Verification items for the finished model (mm, model axes). A direction names the side the tool comes from. Give positions to 0.01 mm unless a question says otherwise; leave off trailing zeros. Loops run counter-clockwise (first coordinate to the right, second up) from the corner with the lowest first, then second, coordinate; pieces in that order, holes last. Notation, with made-up numbers: (81, 33.25) - (86, 33.25) arc R38 cw to (86, 71.25) - close; hole circle Ø1 at (8, 31). An arc over 180 degrees is marked (long way). Put each result on its own line as item: value. Start each with the question number.
```python
from build123d import *

# Parameters (mm, degrees)
SKETCH_1_R          = 1
EXTRUDE_1_DEPTH     = 1.6
SKETCH_2_R          = 1
CUT_EXTRUDE_1_DEPTH = 1.6
EXTRUDE_START       = 1.6
EXTRUDE_2_DEPTH     = 1.6
SKETCH_4_W          = 1.78
SKETCH_4_H          = 8.1
CUT_EXTRUDE_2_DEPTH = 0.1
CUT_EXTRUDE_START   = 1.6
SKETCH_5_W          = 1.78
SKETCH_5_H          = 8.1
CUT_EXTRUDE_3_DEPTH = 0.1
SKETCH_6_W          = 19.5
SKETCH_6_H          = 70
EXTRUDE_3_DEPTH     = 10
CUT_EXTRUDE_START_2 = 40
CUT_EXTRUDE_4_DEPTH = 70
CUT_EXTRUDE_START_3 = -10
SKETCH_9_W          = 19.5
SKETCH_9_H          = 35
CUT_EXTRUDE_5_DEPTH = 4
CUT_EXTRUDE_6_DEPTH = 1.6


with BuildPart() as part:
    # 草图1 → 凸台-拉伸1 (new body)
    with BuildSketch(Plane.XY):
        with BuildLine():
            Line((-14, 50), (14, 50))
            ThreePointArc((14, 50), (15.414213562, 49.414213562), (16, 48))
            Line((16, 48), (16, -48))
            ThreePointArc((16, -48), (15.414213562, -49.414213562), (14, -50))
            Line((14, -50), (-14, -50))
            ThreePointArc((-14, -50), (-15.414213562, -49.414213562), (-16, -48))
            Line((-16, -48), (-16, 48))
            ThreePointArc((-16, 48), (-15.414213562, 49.414213562), (-14, 50))
        make_face()
        with Locations((-14, -48)):
            Circle(SKETCH_1_R, mode=Mode.SUBTRACT)
        with Locations((14, -48)):
            Circle(SKETCH_1_R, mode=Mode.SUBTRACT)
    extrude(amount=EXTRUDE_1_DEPTH)

    # 草图2 → 切除-拉伸1 (cut)
    with BuildSketch(Plane.XY):
        with Locations((-14, 28)):
            Circle(SKETCH_2_R)
        with Locations((14, 28)):
            Circle(SKETCH_2_R)
    extrude(amount=CUT_EXTRUDE_1_DEPTH, mode=Mode.SUBTRACT)

    # 草图3 → 凸台-拉伸2 (add)
    with BuildSketch(Plane.XY.offset(EXTRUDE_START)):
        with BuildLine():
            Line((-7.62, 50), (7.62, 50))
            Line((7.62, 50), (7.62, 59.42))
            ThreePointArc((7.62, 59.42), (7.180660172, 60.480660172), (6.12, 60.92))
            Line((6.12, 60.92), (-6.12, 60.92))
            ThreePointArc((-6.12, 60.92), (-7.180660172, 60.480660172), (-7.62, 59.42))
            Line((-7.62, 59.42), (-7.62, 50))
        make_face()
        with BuildLine():
            Line((-7.62, -59.42), (-7.62, -50))
            Line((-7.62, -50), (7.62, -50))
            Line((7.62, -50), (7.62, -59.42))
            ThreePointArc((7.62, -59.42), (7.180660172, -60.480660172), (6.12, -60.92))
            Line((6.12, -60.92), (-6.12, -60.92))
            ThreePointArc((-6.12, -60.92), (-7.180660172, -60.480660172), (-7.62, -59.42))
        make_face()
    extrude(amount=-EXTRUDE_2_DEPTH)

    # 草图4 → 切除-拉伸2 (cut)
    with BuildSketch(Plane.XY):
        with Locations((0, 56.37)):
            Rectangle(SKETCH_4_W, SKETCH_4_H)
        with Locations((2.54, 56.37)):
            Rectangle(SKETCH_4_W, SKETCH_4_H)
        with Locations((5.08, 56.37)):
            Rectangle(SKETCH_4_W, SKETCH_4_H)
        with Locations((-2.54, 56.37)):
            Rectangle(SKETCH_4_W, SKETCH_4_H)
        with Locations((-5.08, 56.37)):
            Rectangle(SKETCH_4_W, SKETCH_4_H)
        with Locations((-5.08, -56.37)):
            Rectangle(SKETCH_4_W, SKETCH_4_H)
        with Locations((-2.54, -56.37)):
            Rectangle(SKETCH_4_W, SKETCH_4_H)
        with Locations((5.08, -56.37)):
            Rectangle(SKETCH_4_W, SKETCH_4_H)
        with Locations((2.54, -56.37)):
            Rectangle(SKETCH_4_W, SKETCH_4_H)
        with Locations((0, -56.37)):
            Rectangle(SKETCH_4_W, SKETCH_4_H)
    extrude(amount=CUT_EXTRUDE_2_DEPTH, mode=Mode.SUBTRACT)

    # 草图5 → 切除-拉伸3 (cut)
    with BuildSketch(Plane.XY.offset(CUT_EXTRUDE_START)):
        with Locations((2.54, 56.37)):
            Rectangle(SKETCH_5_W, SKETCH_5_H)
        with Locations((0, 56.37)):
            Rectangle(SKETCH_5_W, SKETCH_5_H)
        with Locations((-5.08, 56.37)):
            Rectangle(SKETCH_5_W, SKETCH_5_H)
        with Locations((-2.54, 56.37)):
            Rectangle(SKETCH_5_W, SKETCH_5_H)
        with Locations((5.08, 56.37)):
            Rectangle(SKETCH_5_W, SKETCH_5_H)
        with Locations((2.54, -56.37)):
            Rectangle(SKETCH_5_W, SKETCH_5_H)
        with Locations((5.08, -56.37)):
            Rectangle(SKETCH_5_W, SKETCH_5_H)
        with Locations((-2.54, -56.37)):
            Rectangle(SKETCH_5_W, SKETCH_5_H)
        with Locations((-5.08, -56.37)):
            Rectangle(SKETCH_5_W, SKETCH_5_H)
        with Locations((0, -56.37)):
            Rectangle(SKETCH_5_W, SKETCH_5_H)
    extrude(amount=-CUT_EXTRUDE_3_DEPTH, mode=Mode.SUBTRACT)

    # 草图6 → 凸台-拉伸3 (add)
    with BuildSketch(Plane.XY):
        with Locations((0, 5)):
            Rectangle(SKETCH_6_W, SKETCH_6_H)
    extrude(amount=-EXTRUDE_3_DEPTH)

    # 草图7 → 切除-拉伸4 (cut)
    with BuildSketch(Plane(origin=(0, 0, 0), x_dir=(1, 0, 0), z_dir=(0, 1, 0)).offset(CUT_EXTRUDE_START_2)):
        Polygon((9.75, 10), (9.75, 7), (6.75, 10), align=None)
        Polygon((-9.75, 10), (-6.75, 10), (-9.75, 7), align=None)
    extrude(amount=-CUT_EXTRUDE_4_DEPTH, mode=Mode.SUBTRACT)

    # 草图9 → 切除-拉伸5 (cut)
    with BuildSketch(Plane.XY.offset(CUT_EXTRUDE_START_3)):
        with Locations((0, -12.5)):
            Rectangle(SKETCH_9_W, SKETCH_9_H)
    extrude(amount=CUT_EXTRUDE_5_DEPTH, mode=Mode.SUBTRACT)

    # 草图11 → 切除-拉伸6 (cut)
    with BuildSketch(Plane.XY):
        with BuildLine():
            Line((7.62, -50), (14, -50))
            ThreePointArc((14, -50), (15.414213562, -49.414213562), (16, -48))
            Line((16, -48), (16, -38))
            ThreePointArc((16, -38), (15.414213562, -39.414213562), (14, -40))
            Line((14, -40), (-14, -40))
            ThreePointArc((-14, -40), (-15.414213562, -39.414213562), (-16, -38))
            Line((-16, -38), (-16, -48))
            ThreePointArc((-16, -48), (-15.414213562, -49.414213562), (-14, -50))
            Line((-14, -50), (-7.62, -50))
            Line((-7.62, -50), (-7.62, -59.42))
            ThreePointArc((-7.62, -59.42), (-7.180660172, -60.480660172), (-6.12, -60.92))
            Line((-6.12, -60.92), (6.12, -60.92))
            ThreePointArc((6.12, -60.92), (7.180660172, -60.480660172), (7.62, -59.42))
            Line((7.62, -59.42), (7.62, -50))
        make_face()
    extrude(amount=CUT_EXTRUDE_6_DEPTH, mode=Mode.SUBTRACT)


solid = part.part
```
1) Section check A-A, the plane y = 28. Enter the section's corners in (x, z), plus the area to 3 significant figures.
2) Section check B-B, the plane y = -5. Enter the section's corners in (x, z).
3) Scan lines: line 1 along Y through (x, z) = (14, 0.4); line 2 along Z through (x, y) = (-3.5, -13); line 3 along Z through (x, y) = (0, 47.5). Record each from-to range of solid material in increasing order. Write a range as from..to.
4) Set-up check for faces 1 (the face through (-3, 56, 0.1)), 2 (the face through (11, 50, 1)), 3 (the face through (0, 5, -8)), 4 (the face through (5, 56, 1.5)): record each of +Z, -Z, +X, -X, +Y, -Y from which the full face is reachable in a straight line by a thin tool's end or side.
5) Draft check along X on faces 5 (the face through (8.27, 22.74, -8.48)), 6 (the face through (0, 60.92, 1)), 7 (the face through (0, 56, 0.1)), 8 (the face through (-15.43, 49.4, 0.79)). Enter one of: pulls with the +X half, pulls with the -X half, needs draft (parallel to the pull), parting line crosses it, or undercut.
6) Depth check by flat-ended pin: P1, Ø3, axis at x = -9.5, y = -4.5, coming from the -Z side; P2, Ø4, axis at y = 5, z = -8, coming from the -X side; P3, Ø3, axis at y = -13.5, z = -8.5, coming from the +X side; P4, Ø0.5, axis at y = 56, z = 0.5, coming from the +X side. Enter the tip coordinate at first touch or a pass-through.
Results are:
1. outline: (-16, 0) - (-15, 0) - (-15, 1.6) - (-16, 1.6) - close; (-13, 0) - (-9.75, 0) - (-9.75, -7) - (-6.75, -10) - (6.75, -10) - (9.75, -7) - (9.75, 0) - (13, 0) - (13, 1.6) - (-13, 1.6) - close; (15, 0) - (16, 0) - (16, 1.6) - (15, 1.6) - close
1. area: 231 mm2
2. outline: (-16, 0) - (-9.75, 0) - (-9.75, -6) - (9.75, -6) - (9.75, 0) - (16, 0) - (16, 1.6) - (-16, 1.6) - close
3. line 1: y = -40..27, 29..50
3. line 2: z = -6..1.6
3. line 3: z = 0..1.6
4. face 1: -Z
4. face 2: +Z, -Z, +X, +Y
4. face 3: -Z, +X, -X, -Y
4. face 4: +Z
5. face 5: pulls with the +X half
5. face 6: needs draft
5. face 7: undercut
5. face 8: pulls with the -X half
6. P1: stops at z = -6
6. P2: stops at x = -9.75
6. P3: passes through
6. P4: stops at x = 7.62
